Model file for the job. Use its own axes, mm. Round coordinates to 2 decimals unless told otherwise and drop trailing zeros. Write each loop counter-clockwise with the first axis right and the second up, starting at its lowest first coordinate (ties: lowest second). Pieces come first, ordered by that corner, then holes.
Autodesk Inventor part; units mm, degrees
ref_plane "YZ Plane" through (0, 0, 0) normal (1, 0, 0) x (0, 1, 0)
ref_plane "XZ Plane" through (0, 0, 0) normal (0, 1, 0) x (-1, 0, 0)
ref_plane "XY Plane" through (0, 0, 0) normal (0, 0, 1) x (1, 0, 0)
sketch "スケッチ1" plane through (0, 0, 0) normal (0, 1, 0) x (-1, 0, 0)
  line L0 (0, 0) -> (65.5, 0)
  line L1 (65.5, 0) -> (65.5, -70)
  line L2 (65.5, -70) -> (0, -70)
  line L3 (0, -70) -> (0, 0)
  dimension "d0" = 65.5
  dimension "d1" = 70
extrude "押し出し1" add sketch "スケッチ1" along normal blind 3
sketch "スケッチ3" plane through (0, 3, 0) normal (0, 1, 0) x (1, 0, 0)
  line L0 (-65.5, 0) -> (0, 0)
  line L1 (-32.75, 0) -> (-32.75, 70)
  line L2 (0, 70) -> (-65.5, 70)
  circle A0 centre (-32.75, 35) radius 15.18
  point P0 (-32.75, 50.18)
  point P1 (-45.8963, 42.59)
  point P2 (-45.8963, 27.41)
  point P3 (-32.75, 19.82)
  point P4 (-19.6037, 27.41)
  point P5 (-19.6037, 42.59)
  dimension "d15" = 30.36
  dimension "d18" = 360
hole "穴2" at (-32.75, 3, -50.18) at (-45.8963, 3, -42.59) at (-45.8963, 3, -27.41) at (-32.75, 3, -19.82) at (-19.6037, 3, -27.41) at (-19.6037, 3, -42.59) direction (0, -1, 0) diameter 4.2 end through all
sketch "スケッチ4" plane through (0, 3, 0) normal (0, 1, 0) x (1, 0, 0)
  line L0 (-65.5, 70) -> (-65.5, 0)
  line L1 (0, 70) -> (-65.5, 70)
  circle A0 centre (-32.75, 35) radius 23.5
  line L2 (0, 0) -> (0, 70)
  line L3 (-65.5, 70) -> (0, 70)
  line L4 (0, 70) -> (0, 0)
  line L5 (0, 0) -> (-65.5, 0)
  line L6 (-65.5, 0) -> (-65.5, 70)
  dimension "d27" = 47
  dimension "d28" = 35
  dimension "d29" = 32.75
extrude "押し出し2" cut sketch "スケッチ4" against normal blind 3
sketch "スケッチ5" plane through (-32.75, 3, -35) normal (0, 1, 0) x (1, 0, 0)
  line L0 (58, 30) -> (118, 30)
  line L1 (118, 30) -> (118, -30)
  line L2 (118, -30) -> (58, -30)
  line L3 (58, -30) -> (58, 30)
  circle A0 centre (0, 0) radius 23.5
  line L4 (58, 30) -> (-2.5612, 23.36)
  circle A1 centre (0, 0) radius 23.5
  line L5 (58, -30) -> (-2.5612, -23.36)
  point P0 (32.75, -35)
  point P1 (-2.5612, -23.36)
  dimension "d32" = 60
  dimension "d33" = 60
  dimension "d34" = 30
  dimension "d35" = 58
extrude "押し出し3" add sketch "スケッチ5" against normal blind 3 contours L0 L1 L2 L3 | L3 L5 A0 L4
sketch "スケッチ6" plane through (0, 3, 0) normal (0, 1, 0) x (1, 0, 0)
  line L0 (40.25, 50) -> (70.25, 50)
  line L1 (70.25, 50) -> (70.25, 20)
  line L2 (70.25, 20) -> (40.25, 20)
  line L3 (40.25, 20) -> (40.25, 50)
  line L4 (85.25, 65) -> (25.25, 65)
  point P0 (0, 0)
  dimension "d38" = 30
  dimension "d39" = 30
  dimension "d40" = 15
  dimension "d41" = 15
hole "穴3" at (70.25, 3, -50) at (40.25, 3, -50) at (40.25, 3, -20) at (70.25, 3, -20) direction (0, -1, 0) diameter 4 end through all
properties part number "link3_plate1" material "アルミニウム 6061"
1) Cut at C-C on y = 1.4. Give the number of separate pieces and of enclosed holes in the cut face, and give its area (3 significant figures).
2) Cut at D-D on z = -27.41. List the corners of the cut face in (x, y).
3) Cut at B-B on z = -19.82. List the corners of the cut face in (x, y).
4) Cut at A-A on x = 40.25. List the corners of the cut face in (y, z), and give its area (3 significant figures).
5) Flat gauge pins, fed straight in: pin 1 Ø3.5 at (x, z) = (70.25, -50) entering from +Y; pin 2 Ø1.5 at (x, y) = (-35.5, 2.5) entering from +Z. Where does each tip first touch, or does it go through?
6) Pull direction X, two halves, no side cores. Call faces 1 (the face through (85.25, 2, -35)), 2 (the face through (-45.989, 1.479, -29.508)), 3 (the face through (-4.607, 1.521, -8.274)), 4 (the face through (31, 3, -35)): released by +X, released by -X, zero draft, split by the parting line, or undercut.
7) Wall check: probe 1 along X at (y, z) = (0.8, -44.5); probe 2 along X at (y, z) = (2.05, -19.82); probe 3 along X at (y, z) = (1.3, -27.41). Give the ranges that are in metal, low to high.
Result sheet:
1. separate pieces: 1
1. enclosed holes: 10
1. area: 7,450 mm2
2. outline: (-54.99, 0) - (-48, 0) - (-48, 3) - (-54.99, 3) - close; (-43.8, 0) - (-21.7, 0) - (-21.7, 3) - (-43.8, 3) - close; (-17.5, 0) - (85.25, 0) - (85.25, 3) - (-17.5, 3) - close
3. outline: (-50.69, 0) - (-34.85, 0) - (-34.85, 3) - (-50.69, 3) - close; (-30.65, 0) - (38.26, 0) - (38.26, 3) - (-30.65, 3) - close; (42.24, 0) - (68.26, 0) - (68.26, 3) - (42.24, 3) - close; (72.24, 0) - (85.25, 0) - (85.25, 3) - (72.24, 3) - close
4. outline: (0, -65) - (3, -65) - (3, -52) - (0, -52) - close; (0, -48) - (3, -48) - (3, -22) - (0, -22) - close; (0, -18) - (3, -18) - (3, -5) - (0, -5) - close
4. area: 156 mm2
5. pin 1: passes through
5. pin 2: stops at z = -11.58
6. face 1: released by +X
6. face 2: undercut
6. face 3: released by -X
6. face 4: zero draft
7. probe 1: x = -54.24 to -46.77, -45.02 to -20.48, -18.73 to 85.25
7. probe 2: x = -50.69 to -34.85, -30.65 to 38.26, 42.24 to 68.26, 72.24 to 85.25
7. probe 3: x = -54.99 to -48, -43.8 to -21.7, -17.5 to 85.25
